For this review, use the dimensioned drawing (mm, ordinates from the lowest corner) and the shaded views. A direction names the side the tool comes from. Coordinates: 2 decimals unless noted, no trailing zeros. Loops run counter-clockwise (first coordinate to the right, second up) from the corner with the lowest first, then second, coordinate; pieces in that order, holes last. Notation, with made-up numbers: M 15.5,-19 L 37.5,-19 A23 cw 37.5,15 Z; hole C 17,25.25 d1. An arc over 180 degrees is marked long. Write item = value, one per line. Start each with the question number.
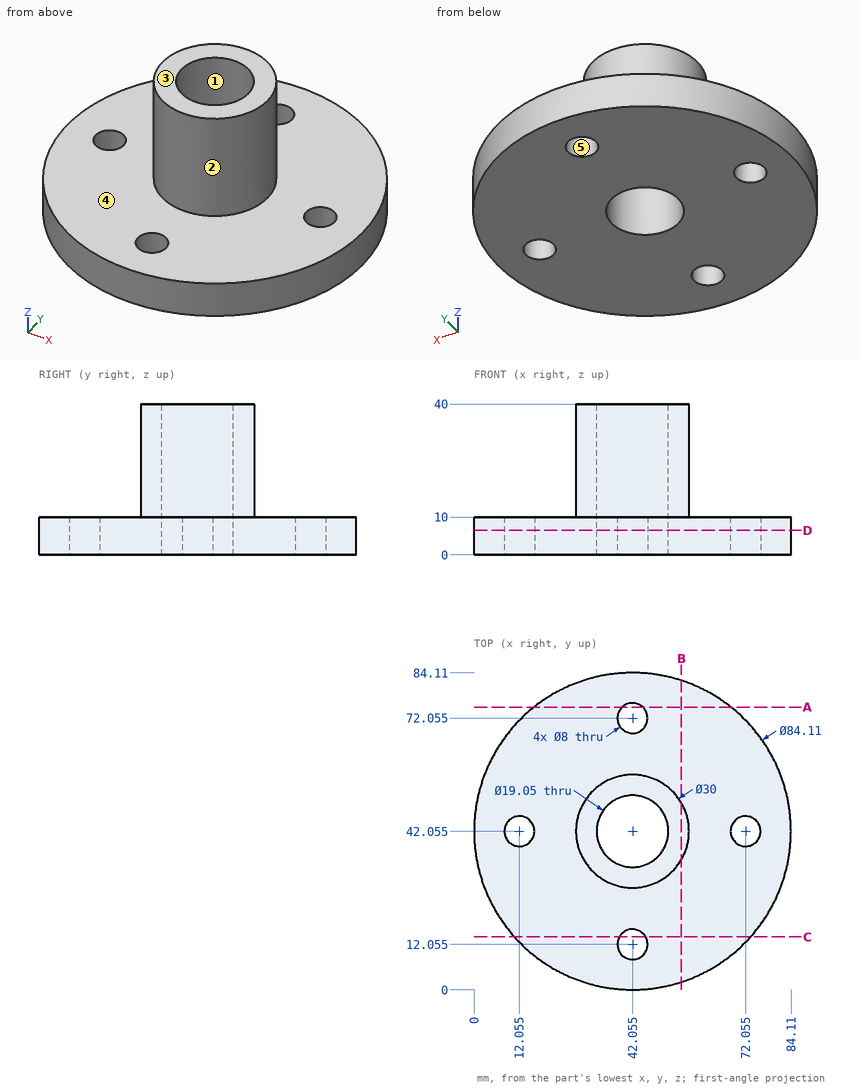
Q1. Add section A-A on y = 75. State the section outline as (x, z) points, plus the area to 3 significant figures.
Q2. For the marked faces 4 and 5, list the 3-axis set-ups (+Z, -Z, +X, -X, +Y, -Y) from which the entire face can be reached by the end or side of a thin tool; tool diameter is ignored.
Q3. Mouldability with a two-part tool opening along X and no side actions: class the marked faces 1, 2 and 3 as released by +X, released by -X, zero draft, split by the parting line, or undercut.
Q4. Clearance check with flat-ended pins moving along their axes: P1, Ø7, axis at x = 42.055, y = 72.055, coming from the +Z side; P2, Ø10, axis at y = 32, z = 31, coming from the +X side; P3, Ø8, axis at x = 21, y = 51.5, coming from the +Z side; P4, Ø8, axis at x = 30, z = 18.5, coming from the +Y side. State where each tip first meets the part, or that it passes through.
Q5. Add section D-D on z = 6.5. State the section outline as (x, y) points (3 decimals), plus the area to 3 significant figures.
Q6. Add section B-B on x = 55. State the section outline as (y, z) points.
Q7. To check wall thickness, follow line 1 (X direction, y = 42.5, z = 19); line 2 (Z direction, x = 53, y = 7.5); line 3 (Y direction, x = 46, z = 22). State the ranges of each line that lie inside material, in increasing order. Write a range as from..to.
Q8. Add section C-C on y = 14. State the section outline as (x, z) points, plus the area to 3 significant figures.
Values follow:
q1.outline = M 15.92,0 L 39.35,0 L 39.35,10 L 15.92,10 Z; M 44.76,0 L 68.19,0 L 68.19,10 L 44.76,10 Z
q1.area = 469 mm2
q2.face_4 = +Z
q2.face_5 = +Z, -Z
q3.face_1 = undercut
q3.face_2 = split by the parting line
q3.face_3 = zero draft
q4.P1 = through
q4.P2 = 56.18
q4.P3 = 10
q4.P4 = 54.71
q5.outline = C 42.055,42.055 d84.11; hole C 12.055,42.055 d8; hole C 42.055,42.055 d19.05; hole C 42.055,12.055 d8; hole C 42.055,72.055 d8; hole C 72.055,42.055 d8
q5.area = 5,070 mm2
q6.outline = M 2.04,0 L 82.07,0 L 82.07,10 L 49.63,10 L 49.63,40 L 34.48,40 L 34.48,10 L 2.04,10 Z
q7.line_1 = 27.06..32.54, 51.57..57.05
q7.line_2 = 0..10
q7.line_3 = 27.58..33.39, 50.72..56.53
q8.outline = M 10.73,0 L 38.56,0 L 38.56,10 L 10.73,10 Z; M 45.55,0 L 73.38,0 L 73.38,10 L 45.55,10 Z
q8.area = 557 mm2
